For this review, take the finished solid that the model builds, in its own axes (mm). Face numbers are marked on the shaded views. Round coordinates to 2 decimals unless told otherwise and drop trailing zeros. Loops run counter-clockwise (first coordinate to the right, second up) from the corner with the lowest first, then second, coordinate; pieces in that order, holes last.
1) Take a section at A-A (z = 1). State the section outline as (x, y) points.
2) Take a section at B-B (y = 3.5). State the section outline as (x, z) points, then the cut area to 3 significant figures.
3) Take a section at D-D (x = 33). State the section outline as (y, z) points, then the cut area to 3 significant figures.
4) Insertion check: pin 1 (4 mm diameter, centred on x = 44, y = 3.5, fed in from +Z); pin 2 (3 mm diameter, centred on x = 46, z = 0, fed in from -Y); pin 3 (3 mm diameter, centred on y = 3.5, z = -1.5, fed in from -X); pin 4 (3 mm diameter, centred on x = -7, y = 2.5, fed in from -Z). Each pin has a flat end and moves straight along its axis. Give the tip position at first contact, or say it passes through.
5) Mouldability with a two-part tool opening along X and no side actions: class the marked faces 1, 2 and 3 as pulls with the +X half, pulls with the -X half, needs draft (parallel to the pull), parting line crosses it, or undercut.
6) Wall thickness on L1, parallel to X at y = 4, z = -5.25; L2, parallel to X at y = 1.25, z = -5.75; L3, parallel to Z at x = 46.5, y = 4.25: over which ranges is each line inside the solid? List them lowest first.
7) Take a section at C-C (z = -3.25). State the section outline as (x, y) points, then the cut area to 3 significant figures.
```python
from build123d import *

# Parameters (mm, degrees)
BOSS_EXTRUDE1_DEPTH = 7.62


with BuildPart() as part:
    # Sketch2 → Boss-Extrude1 (new body)
    with BuildSketch(Plane(origin=(0, 0, 0), x_dir=(1, 0, 0), z_dir=(0, 1, 0))):
        with BuildLine():
            ThreePointArc((87.481333576, -5.178289999), (98.907220268, -9.79891701), (106.382667152, 0))
            Line((106.382667152, 0), (103.555015571, 0))
            Line((103.555015571, 0), (101.721928466, -3.175))
            Line((101.721928466, -3.175), (99.888841361, -6.35))
            Line((99.888841361, -6.35), (92.556492943, -6.35))
            Line((92.556492943, -6.35), (90.723405838, -3.175))
            Line((90.723405838, -3.175), (88.890318733, 0))
            Line((88.890318733, 0), (0, 0))
            Line((0, 0), (-3.81, -6.35))
            Line((-3.81, -6.35), (-10.16, -6.35))
            Line((-10.16, -6.35), (-10.16, -7.931147458))
            ThreePointArc((-10.16, -7.931147458), (-1.986767948, -9.995070029), (4.931333576, -5.178289999))
            Line((4.931333576, -5.178289999), (87.481333576, -5.178289999))
        make_face()
        with BuildLine():
            Line((87.481333576, 5.178289999), (4.931333576, 5.178289999))
            ThreePointArc((4.931333576, 5.178289999), (-1.986767948, 9.995070029), (-10.16, 7.931147458))
            Line((-10.16, 7.931147458), (-10.16, 6.35))
            Line((-10.16, 6.35), (-3.81, 6.35))
            Line((-3.81, 6.35), (0, 0))
            Line((0, 0), (88.890318733, 0))
            Line((88.890318733, 0), (92.556492943, 6.35))
            Line((92.556492943, 6.35), (99.888841361, 6.35))
            Line((99.888841361, 6.35), (103.555015571, 0))
            Line((103.555015571, 0), (106.382667152, 0))
            ThreePointArc((106.382667152, 0), (98.907220268, 9.79891701), (87.481333576, 5.178289999))
        make_face()
    extrude(amount=BOSS_EXTRUDE1_DEPTH)


solid = part.part
```
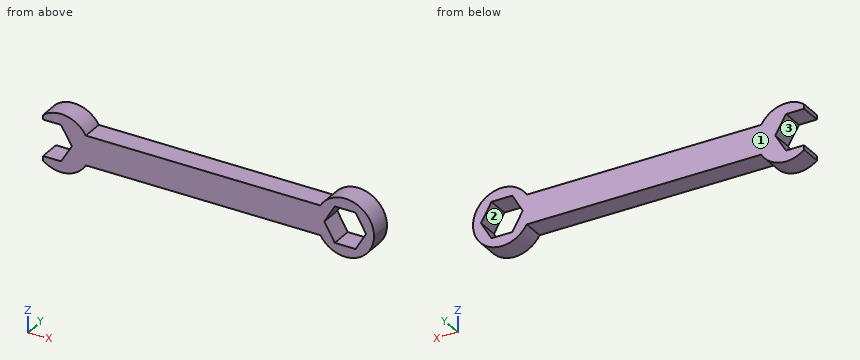
Response:
1. outline: (-0.6, 0) - (89.47, 0) - (89.47, 7.62) - (-0.6, 7.62) - close; (102.98, 0) - (106.33, 0) - (106.33, 7.62) - (102.98, 7.62) - close
2. outline: (-10.16, -7.93) arc R10.16 ccw to (4.93, -5.18) - (87.48, -5.18) arc R10.16 ccw (long way) to (87.48, 5.18) - (4.93, 5.18) arc R10.16 ccw to (-10.16, 7.93) - (-10.16, 6.35) - (-3.81, 6.35) - (0, 0) - (-3.81, -6.35) - (-10.16, -6.35) - close; hole (88.89, 0) - (92.56, -6.35) - (99.89, -6.35) - (103.56, 0) - (99.89, 6.35) - (92.56, 6.35) - close
2. area: 1,200 mm2
3. outline: (0, -5.18) - (7.62, -5.18) - (7.62, 5.18) - (0, 5.18) - close
3. area: 78.9 mm2
4. pin 1: stops at z = 5.18
4. pin 2: stops at y = 0
4. pin 3: stops at x = -1.8
4. pin 4: stops at z = -10.02
5. face 1: needs draft
5. face 2: undercut
5. face 3: pulls with the -X half
6. L1: x = -3.15 to 4.89, 87.52 to 91.92, 100.52 to 104.92
6. L2: x = -3.45 to 4.57, 87.85 to 92.21, 100.24 to 104.6
6. L3: z = -5.18 to 5.18
7. outline: (-1.95, 0) - (90.77, 0) - (90.77, 7.62) - (-1.95, 7.62) - close; (101.68, 0) - (105.85, 0) - (105.85, 7.62) - (101.68, 7.62) - close
7. area: 738 mm2
